Autodesk Inventor part; units mm, degrees
ref_plane "YZ Plane" through (0, 0, 0) normal (1, 0, 0) x (0, 1, 0)
ref_plane "XZ Plane" through (0, 0, 0) normal (0, 1, 0) x (-1, 0, 0)
ref_plane "XY Plane" through (0, 0, 0) normal (0, 0, 1) x (1, 0, 0)
sketch "Sketch1" plane through (0, 0, 0) normal (1, 0, 0) x (0, 1, 0)
  line L0 (7.8254, 10.5896) -> (-4.8746, 10.5896)
  line L1 (-4.8746, 10.5896) -> (-4.8746, -8.4604)
  line L2 (-4.8746, -8.4604) -> (7.8254, -8.4604)
  line L3 (7.8254, -8.4604) -> (7.8254, 10.5896)
  point P0 (0, 0)
  dimension "d0" = 19.05
  dimension "d1" = 12.7
extrude "Extrusion1" add sketch "Sketch1" along normal blind 27.94
sketch "Sketch2" plane through (27.94, 0, 0) normal (1, 0, 0) x (0, 0, -1)
  line L0 (-10.5896, 7.8254) -> (-10.5896, -4.8746)
  line L1 (8.4604, 7.8254) -> (-10.5896, 7.8254)
  point P0 (0, 0)
  point P1 (-4.2396, 1.4754)
  dimension "d4" = 6.35
  dimension "d5" = 6.35
hole "Hole1" at (27.94, 1.4754, 4.2396) direction (-1, 0, 0) diameter 4.318 end through all
sketch "Sketch3" plane through (0, 7.8254, 10.5896) normal (0, 1, 0) x (1, 0, 0)
  line L0 (27.94, 19.05) -> (27.94, 0)
  line L1 (0, 19.05) -> (0, 0)
  line L2 (0, 19.05) -> (27.94, 19.05)
  point P0 (0, 10.5896)
  point P1 (6.35, 12.7)
  point P2 (21.59, 12.7)
  dimension "d13" = 6.35
  dimension "d14" = 6.35
  dimension "d15" = 6.35
  dimension "d16" = 0
hole "Hole2" at (6.35, 7.8254, -2.1104) at (21.59, 7.8254, -2.1104) direction (0, -1, 0) diameter 4.318 end through all
properties part number "MotorSpacerBlock"
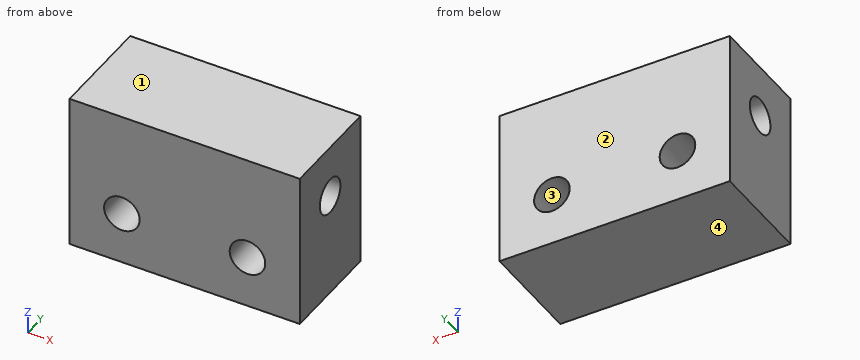
Model file for the job. Use its own axes, mm. Face numbers are marked on the shaded views. Coordinates: 2 decimals unless noted, no trailing zeros. Loops run counter-clockwise (first coordinate to the right, second up) from the corner with the lowest first, then second, coordinate; pieces in that order, holes last. Notation, with made-up numbers: (-1.75, -25) -> (17.25, -25) arc R10 ccw to (17.25, -15) -> close; hole circle Ø11 at (20.25, 82). An arc over 180 degrees is marked (long way). Use one line per item in the form item = value. Start each with the question number.
(1) Cut at C-C on x = 23. Give the cut face in (y, z), and give its area (3 significant figures).
(2) Flat gauge pin, fed straight in: pin 1 (4 mm diameter, centred on x = 6.35, z = -2.11, fed in from +Y). Where does the tip first touch, or does it go through?
(3) Cut at A-A on x = 5. Give the cut face in (y, z).
(4) Probe probe 1 along X at (y, z) = (6.25, -2.25); probe 2 along Z at (x, y) = (21.59, 4); probe 3 along X at (y, z) = (5.75, -4). List the from-to ranges inside material, lowest first. Write a range as from..to.
(5) Cut at B-B on y = 2.5. Give the cut face in (x, z).
(6) Cut at D-D on y = 6.25. Give the cut face in (x, z), and give its area (3 significant figures).
(7) Pull direction Z, two halves, no side cores. Call the marked faces 1, 2, 3 and 4: pulls with the +Z half, pulls with the -Z half, needs draft (parallel to the pull), parting line crosses it, or undercut.
Values:
q1.outline = (-4.87, -8.46) -> (7.83, -8.46) -> (7.83, -3.75) -> (-4.87, -3.75) -> close; (-4.87, -0.48) -> (7.83, -0.48) -> (7.83, 10.59) -> (-4.87, 10.59) -> close; hole circle Ø4.32 at (1.48, 4.24)
q1.area = 186 mm2
q2.pin_1 = through
q3.outline = (-4.87, -8.46) -> (7.83, -8.46) -> (7.83, -3.8) -> (-4.87, -3.8) -> close; (-4.87, -0.43) -> (7.83, -0.43) -> (7.83, 10.59) -> (-4.87, 10.59) -> close; hole circle Ø4.32 at (1.48, 4.24)
q4.probe_1 = 0..4.2, 8.5..19.44, 23.74..27.94
q4.probe_2 = -8.46..-4.27, 0.05..10.59
q4.probe_3 = 0..5.31, 7.39..20.55, 22.63..27.94
q5.outline = (0, -8.46) -> (27.94, -8.46) -> (27.94, 2.34) -> (0, 2.34) -> close; (0, 6.14) -> (27.94, 6.14) -> (27.94, 10.59) -> (0, 10.59) -> close; hole circle Ø4.32 at (6.35, -2.11); hole circle Ø4.32 at (21.59, -2.11)
q6.outline = (0, -8.46) -> (27.94, -8.46) -> (27.94, 10.59) -> (0, 10.59) -> close; hole circle Ø4.32 at (6.35, -2.11); hole circle Ø4.32 at (21.59, -2.11)
q6.area = 503 mm2
q7.face_1 = pulls with the +Z half
q7.face_2 = needs draft
q7.face_3 = undercut
q7.face_4 = pulls with the -Z half
